from build123d import *

# Parameters (mm, degrees)
SKETCH1_R                        = 48
SKETCH1_R_2                      = 8
EX_CARRIER_FRONT_PLATE_4MM_DEPTH = 2
SKETCH2_R                        = 6
CUT_PIN_HOLE_12_DEPTH            = 69
PAT_PIN_HOLES_3X120_COUNT        = 3
CUT_EXTRUDE1_DEPTH               = 1
SKETCH4_R                        = 2.75
CUT_EXTRUDE2_DEPTH               = 68.911707385
SKETCH5_R                        = 2.75
CUT_EXTRUDE3_DEPTH               = 68.911707385
CIRPATTERN1_COUNT                = 3
CIRPATTERN2_COUNT                = 3


with BuildPart() as part:
    # Sketch1 → EX_Carrier_Front_Plate_4mm (new, symmetric)
    with BuildSketch(Plane.XY):
        Circle(SKETCH1_R)
        Circle(SKETCH1_R_2, mode=Mode.SUBTRACT)
    extrude(amount=EX_CARRIER_FRONT_PLATE_4MM_DEPTH, both=True)

    # Sketch2 → CUT_Pin_Hole_Ø12 (cut, symmetric)
    with BuildSketch(Plane.XY.offset(2)):
        with Locations((0, 33.75)):
            Circle(SKETCH2_R)
    cut_pin_hole_12 = extrude(amount=CUT_PIN_HOLE_12_DEPTH, both=True, mode=Mode.SUBTRACT)

    # PAT_Pin_Holes_3x120: CUT_Pin_Hole_Ø12 ×3 about axis
    pat_pin_holes_3x120_axis = Axis((0, 0, 0), (0, 0, 1))
    for i in range(1, PAT_PIN_HOLES_3X120_COUNT):
        add(cut_pin_hole_12.rotate(pat_pin_holes_3x120_axis, i * 360 / PAT_PIN_HOLES_3X120_COUNT), mode=Mode.SUBTRACT)

    # Sketch3 → Cut-Extrude1 (cut, symmetric)
    with BuildSketch(Plane(origin=(0, 0, 0), x_dir=(0, 0, -1), z_dir=(1, 0, 0))):
        Polygon((-2, 44.889744608), (0, 48), (-2, 48), align=None)
    extrude(amount=CUT_EXTRUDE1_DEPTH, both=True, mode=Mode.SUBTRACT)

    # Sketch4 → Cut-Extrude2 (cut, through all)
    with BuildSketch(Plane.XY):
        with Locations((0, -33.75)):
            Circle(SKETCH4_R)
    cut_extrude2 = extrude(amount=CUT_EXTRUDE2_DEPTH, mode=Mode.SUBTRACT)

    # Sketch5 → Cut-Extrude3 (cut, through all)
    with BuildSketch(Plane.XY):
        with Locations((0, -33.75)):
            Circle(SKETCH5_R)
    cut_extrude3 = extrude(amount=-CUT_EXTRUDE3_DEPTH, mode=Mode.SUBTRACT)

    # CirPattern1: Cut-Extrude2 ×3 about axis
    cirpattern1_axis = Axis((0, 0, 0), (0, 0, 1))
    for i in range(1, CIRPATTERN1_COUNT):
        add(cut_extrude2.rotate(cirpattern1_axis, i * 360 / CIRPATTERN1_COUNT), mode=Mode.SUBTRACT)

    # CirPattern2: Cut-Extrude3 ×3 about axis
    cirpattern2_axis = Axis((0, 0, -2.208265016), (0, 0, 1))
    for i in range(1, CIRPATTERN2_COUNT):
        add(cut_extrude3.rotate(cirpattern2_axis, i * 360 / CIRPATTERN2_COUNT), mode=Mode.SUBTRACT)


solid = part.part
Could you check a few things on this model? Use its own coordinates, in mm. Give positions to 0.01 mm unless a question says otherwise; leave off trailing zeros. Order: outer loops, then holes, each group sorted by start corner. A loop starts at its lowest first (then second) coordinate and runs counter-clockwise, first axis right, second up. Notation, with made-up numbers: (-22.75, 87) - (-6.75, 87) arc R37 cw to (-6.75, 124) - close; hole circle Ø3 at (12, -4). An arc over 180 degrees is marked (long way). Return JSON: item names as keys, results as strings. Group by question number.
Q1. Thinking about a two-plate mould opening in X: for faces 1 (the face through (10, 1, 2)), 2 (the face through (-1.301, 27.893, 0.028)), 3 (the face through (-47.954, 2.11, 0.028)), which applies, pulls with the +X half, pulls with the -X half, needs draft (parallel to the pull), parting line crosses it, or undercut?
Q2. Suppose I cut it at C-C, the plane z = 1.35. Please give me the cut outline in (x, y) (3 decimals), and give its area (3 significant figures).
Q3. Suppose I cut it at A-A, the plane y = 0. Please give me the cut outline in (x, z).
Q4. Please list where these lines run through material, in increasing order: line 1 along Y through (x, z) = (0, -0.55); line 2 along Y through (x, z) = (29, 0); line 3 along X through (y, z) = (-13, 1.7). Write a range as [from, to].
Q5. Will these pins go through, and if not, where does the flat tip stop? pin 1 Ø4.5 at (x, y) = (0, -33.75) entering from -Z; pin 2 Ø1 at (y, z) = (13.5, 0) entering from +X; pin 3 Ø1 at (y, z) = (18.5, 0) entering from +X.
Q6. Suppose I cut it at D-D, the plane x = -10. Please give me the cut outline in (y, z).
Q7. Suppose I cut it at B-B, the plane x = 25. Please give me the cut outline in (y, z), and give its area (3 significant figures).
Resolved:
{
 "1": {"face 1": "needs draft", "face 2": "undercut", "face 3": "parting line crosses it"},
 "2": {"outline": "(-1, 45.901) - (-1, 47.99) arc R48 ccw (long way) to (1, 47.99) - (1, 45.901) - close; hole circle Ø12 at (-29.228, -16.875); hole circle Ø5.5 at (-29.228, 16.875); hole circle Ø16 at (0, 0); hole circle Ø12 at (0, 33.75); hole circle Ø5.5 at (0, -33.75); hole circle Ø12 at (29.228, -16.875); hole circle Ø5.5 at (29.228, 16.875)", "area": "6,620 mm2"},
 "3": {"outline": "(-48, -2) - (-8, -2) - (-8, 2) - (-48, 2) - close; (8, -2) - (48, -2) - (48, 2) - (8, 2) - close"},
 "4": {"line 1": "y = [-48, -36.5], [-31, -8], [8, 27.75], [39.75, 48]", "line 2": "y = [-38.25, -22.87], [-10.88, 14.13], [19.62, 38.25]", "line 3": "x = [-46.21, -33.81], [-24.65, 24.65], [33.81, 46.21]"},
 "5": {"pin 1": "passes through", "pin 2": "stops at x = 46.21", "pin 3": "stops at x = 44.5"},
 "6": {"outline": "(-46.95, -2) - (46.95, -2) - (46.95, 2) - (-46.95, 2) - close"},
 "7": {"outline": "(-40.98, -2) - (-21.13, -2) - (-21.13, 2) - (-40.98, 2) - close; (-12.62, -2) - (40.98, -2) - (40.98, 2) - (-12.62, 2) - close", "area": "294 mm2"}
}
